```python
from build123d import *

# Parameters (mm, degrees)
F1_DEPTH = 63.5
F2_DEPTH = 25.4
F3_DEPTH = 12.7
F4_W     = 19.1736370325
F4_H     = 18.7656953931
F5_DEPTH = 25.4
F8_DEPTH = 24.384


with BuildPart() as f1:
    # F0 (on Front) → F1 (new body, symmetric)
    with BuildSketch(Plane.XZ):
        Polygon((43.002218008, -9.3683367595), (43.002218008, 9.3683367595), (23.952218008, 9.3683367595), (-43.002218008, 9.3683367595), (-43.002218008, -9.3683367595), align=None)
    extrude(amount=F1_DEPTH, both=True)

    # F0 (on Front) → F2 (join, symmetric)
    with BuildSketch(Plane.XZ):
        with BuildLine():
            Line((23.952218008, 9.3683367595), (43.002218008, 9.3683367595))
            Line((43.002218008, 9.3683367595), (43.002218008, 47.7631762624))
            ThreePointArc((43.002218008, 47.7631762624), (45.4664077762, 53.712256621), (51.4154881348, 56.1764463891))
            Line((51.4154881348, 56.1764463891), (56.8243600428, 56.1764463891))
            Line((56.8243600428, 56.1764463891), (56.8243600428, 75.2264463891))
            Line((56.8243600428, 75.2264463891), (51.4154881348, 75.2264463891))
            add(Edge.make_bspline(
                [(41.8041992357, 73.4897059886), (45.002733463, 74.1877892991), (48.2117770705, 74.7703432953), (51.4154881348, 75.2264463891)],
                knots=[107.1334915157, 107.1334915157, 107.1334915157, 107.1334915157, 115.1173046821, 115.1173046821, 115.1173046821, 115.1173046821], degree=3))
            ThreePointArc((41.8041992357, 73.4897059886), (28.8523696739, 63.4200243288), (23.952218008, 47.7631762624))
            Line((23.952218008, 47.7631762624), (23.952218008, 9.3683367595))
        make_face()
    extrude(amount=F2_DEPTH, both=True)

    # F0 (on Front) → F3 (join, symmetric)
    with BuildSketch(Plane.XZ):
        with BuildLine():
            Line((-43.002218008, 9.3683367595), (23.952218008, 9.3683367595))
            Line((23.952218008, 9.3683367595), (23.952218008, 47.7631762624))
            ThreePointArc((23.952218008, 47.7631762624), (28.8523696739, 63.4200243288), (41.8041992357, 73.4897059886))
            add(Edge.make_bspline(
                [(-43.002218008, 9.3683367595), (-42.1446492068, 33.9519638821), (-1.1164118011, 64.1222394823), (41.8041992357, 73.4897059886)],
                knots=[0, 0, 0, 0, 107.1334915157, 107.1334915157, 107.1334915157, 107.1334915157], degree=3))
        make_face()
    extrude(amount=F3_DEPTH, both=True)

    # F4 (on Front) → F5 (join, symmetric)
    with BuildSketch(Plane.XZ):
        with Locations((66.3682073355, 65.5188672245)):
            Rectangle(F4_W, F4_H)
    extrude(amount=F5_DEPTH, both=True)

    # F7 (on face) → F8 (join)
    with BuildSketch(Plane.XY.offset(74.901714921)):
        with BuildLine():
            ThreePointArc((74.5427201599, -25.4), (94.0875248733, -18.8547135488), (102.4145857599, 0))
            ThreePointArc((102.4145857599, 0), (94.0875248733, 18.8547135488), (74.5427201599, 25.4))
            Line((74.5427201599, 25.4), (75.9550258517, 25.4))
            Line((75.9550258517, 25.4), (75.9550258517, -25.4))
            Line((75.9550258517, -25.4), (74.5427201599, -25.4))
        make_face()
    extrude(amount=-F8_DEPTH)


solid = f1.part
```
Work out the finished part from the listing and answer in its coordinate system (mm). A direction names the side the tool comes from. Round coordinates to 2 decimals unless told otherwise and drop trailing zeros. Write each loop counter-clockwise with the first axis right and the second up, starting at its lowest first coordinate (ties: lowest second). Pieces come first, ordered by that corner, then holes. Notation, with made-up numbers: (17.5, -3.5) -> (48.5, -3.5) arc R21 cw to (48.5, 12.5) -> close; hole circle Ø5 at (28, 30). An arc over 180 degrees is marked (long way). Write each question's results on one line, items separated by ' | '.
Q1. Straight lines are drawn through the part: line 1 along X through (y, z) = (23.5, 27); line 2 along Z through (x, y) = (57, 14); line 3 along Y through (x, z) = (3, 36.5). For each, find the intervals that lie inside material, in ascending order. Write a range as [from, to].
Data:
line 1: [23.95, 43] | line 2: [56.14, 74.9] | line 3: [-12.7, 12.7]
Q2. Determine the mould class of faces 4 (the cylindrical face through (45.401, -0.356, 53.646)), 5 (the flat face through (23.952, 19, 29)), 6 (the flat face through (43.002, -1, 12)), 7 (the flat face through (1, 38, 9.368)) for opening direction X: released by +X, released by -X, zero draft, split by the parting line, or undercut.
Data:
face 4: undercut | face 5: released by -X | face 6: released by +X | face 7: zero draft
Q3. Which of the six approach directions +Z, -Z, +X, -X, +Y, -Y give full straight-line access (tool end or side, diameter ignored) to faces 1 (the cylindrical face through (28.986, 18.961, 63.611)), 2 (the flat face through (54, 0, 56.176)), 3 (the flat face through (1, -38, 9.368))?
Data:
face 1: +Z, -X, +Y | face 2: -Z, +Y, -Y | face 3: +Z, -X, -Y
Q4. Section A-A, the plane y = -44 is taken. Write down the section's boundary in (x, z).
Data:
outline: (-43, -9.37) -> (43, -9.37) -> (43, 9.37) -> (-43, 9.37) -> close
Q5. Section B-B, the plane x = 87.5 is taken. Write down the section's boundary in (y, z), then the cut area to 3 significant figures.
Data:
outline: (-23.21, 50.52) -> (23.21, 50.52) -> (23.21, 74.9) -> (-23.21, 74.9) -> close | area: 1,130 mm^2
Q6. Flat-ended cylindrical pins translate along their axes: P1, Ø4, axis at y = 10.5, z = 12, coming from the -X side; P2, Ø8.5, axis at x = 84, y = 12, coming from the -Z side; P3, Ø5, axis at y = 23.5, z = 52.5, coming from the -X side. Find the tip coordinate at first contact, or state that the pin passes through.
Data:
P1: x = -42.97 | P2: z = 50.52 | P3: x = 24.04
